Check sheet for the modelled part. Datum: model origin and axes. Units: mm. Round coordinates to 2 decimals unless told otherwise and drop trailing zeros. Write each loop counter-clockwise with the first axis right and the second up, starting at its lowest first coordinate (ties: lowest second). Pieces come first, ordered by that corner, then holes. Notation, with made-up numbers: (36.5, -24) - (50.5, -24) arc R21 cw to (50.5, -7) - close; hole circle Ø1 at (-38.75, 2.5). An arc over 180 degrees is marked (long way). Answer as a JSON object with one key per item and string values. Group by question number.
Item 1: Sectioned sample at A-A on y = -63. Record the boundary of the cut face in (x, z).
Item 2: Gauge pin test, flat ends, axial feed: P1, Ø1.5, axis at y = -98, z = 2, coming from the -X side; P2, Ø0.9, axis at x = 34.5, z = 1, coming from the -Y side. Record the tip position at first contact, or that the pin passes through.
Item 3: Thickness scan on line 1 (X direction, y = -71, z = 1.25); line 2 (X direction, y = -133, z = 1.75); line 3 (Y direction, x = 62, z = 2.3). Record the ranges inside material, lowest first.
Item 4: Sectioned sample at D-D on y = -9.5. Record the boundary of the cut face in (x, z), plus the area to 3 significant figures.
Item 5: Sectioned sample at C-C on z = 1.75. Record the boundary of the cut face in (x, y), plus the area to 3 significant figures.
Item 6: Sectioned sample at B-B on x = 58. Record the boundary of the cut face in (y, z), plus the area to 3 significant figures.
Autodesk Fusion 360 part; units mm, degrees
sketch "Sketch1" plane through (0, 0, 0) normal (0, 0, 1) x (1, 0, 0)
  line L0 (0, 0) -> (70, 0)
  line L1 (70, 0) -> (70, 70)
  line L2 (70, 70) -> (0, 70)
  line L3 (0, 70) -> (0, 0)
  line L4 (70, 0) -> (55, 0)
  line L5 (0, 0) -> (15, 0)
  line L6 (15, 0) -> (15, -100)
  line L7 (55, 0) -> (55, -100)
  line L8 (55, -100) -> (70, -100)
  line L9 (15, -100) -> (0, -100)
  line L10 (0, -100) -> (0, -145)
  line L11 (70, -100) -> (70, -145)
  line L12 (70, -145) -> (0, -145)
  line L13 (35, -145) -> (36.55, -145)
  line L14 (35, -145) -> (33.45, -145)
  line L15 (36.55, -145) -> (36.55, -45)
  line L16 (33.45, -145) -> (33.45, -45)
  line L17 (33.45, -45) -> (36.55, -45)
  dimension "d1" = 70
  dimension "d2" = 70
  dimension "d3" = 15
  dimension "d4" = 15
  dimension "d5" = 100
  dimension "d6" = 100
  dimension "d7" = 15
  dimension "d8" = 15
  dimension "d9" = 45
  dimension "d10" = 45
  dimension "d11" = 1.55
  dimension "d12" = 1.55
  dimension "d13" = 100
  dimension "d14" = 100
  dimension "d17" = 33.25
  dimension "d18" = 33.25
extrude "Extrude1" add sketch "Sketch1" along normal blind 3 contours L0 L1 L2 L3 L4 L5 | L0 L6 L7 L8 L9 L10 L11 L12 L15 L16 L17
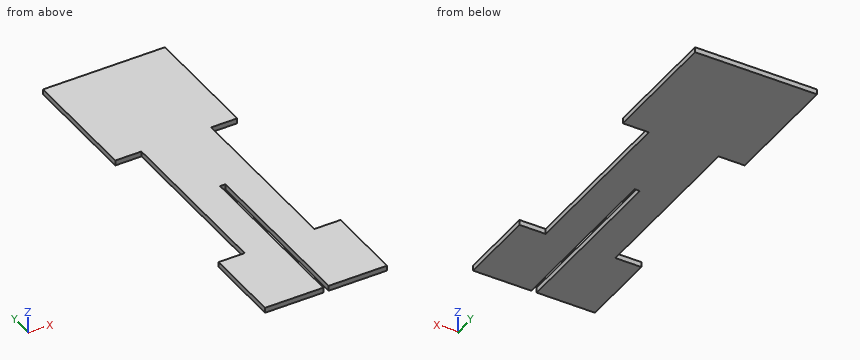
Completed:
{
 "1": {"outline": "(15, 0) - (33.45, 0) - (33.45, 3) - (15, 3) - close; (36.55, 0) - (55, 0) - (55, 3) - (36.55, 3) - close"},
 "2": {"P1": "x = 15", "P2": "y = -45"},
 "3": {"line 1": "15 to 33.45, 36.55 to 55", "line 2": "0 to 33.45, 36.55 to 70", "line 3": "-145 to -100, 0 to 70"},
 "4": {"outline": "(15, 0) - (55, 0) - (55, 3) - (15, 3) - close", "area": "120 mm²"},
 "5": {"outline": "(0, -145) - (33.45, -145) - (33.45, -45) - (36.55, -45) - (36.55, -145) - (70, -145) - (70, -100) - (55, -100) - (55, 0) - (70, 0) - (70, 70) - (0, 70) - (0, 0) - (15, 0) - (15, -100) - (0, -100) - close", "area": "11,700 mm²"},
 "6": {"outline": "(-145, 0) - (-100, 0) - (-100, 3) - (-145, 3) - close; (0, 0) - (70, 0) - (70, 3) - (0, 3) - close", "area": "345 mm²"}
}
